Geometry: final body of the model. Coordinates: model frame, mm. Face numbers are marked on the shaded views. A direction names the side the tool comes from. Give positions to 0.01 mm unless a question says otherwise; leave off trailing zeros. Write each loop counter-clockwise with the first axis right and the second up, starting at its lowest first coordinate (ties: lowest second). Pieces come first, ordered by that corner, then holes. Notation, with made-up numbers: M -37.5,-15 L 12.5,-15 A22 cw 12.5,-1 Z; hole C 45.25,-14.5 d7. An arc over 180 degrees is marked long. Use a Markdown table: item, result. Add a question column.
(1) Pin query (flat end, axial travel): pin 1 Ø0.9 at (x, z) = (16.5, 5.5) entering from -Y; pin 2 Ø6 at (x, y) = (12.5, 1) entering from +Z (3 decimals); pin 3 Ø8 at (x, y) = (-6.5, 0) entering from +Z; pin 4 Ø8.5 at (x, y) = (9, 0) entering from +Z. Return the tip coordinate at first contact, or that it passes through.
(2) Material intervals for L1, parallel to Y at x = 9, z = 1; L2, parallel to X at y = -2, z = 3.25 (3 decimals); L3, parallel to Z at x = -6, y = 5, sorted ascending.
(3) Cut plane B-B (z = 4.25). Output: boundary loops of the cut face in (x, y) (3 decimals).
(4) Draft query along X for the marked faces 4, 5 and 6. Return one class per face: released by +X, released by -X, zero draft, split by the parting line, or undercut.
(5) Cut plane C-C (x = 9). Output: boundary loops of the cut face in (y, z).
(6) Cut plane D-D (y = 2.5). Output: boundary loops of the cut face in (x, z) (3 decimals).
(7) Reachability of the marked faces 1, 2 and 3 from +Z, -Z, +X, -X, +Y, -Y: full face, straight path, thin tool, end or side. Return the list, or none.
(8) Cut plane A-A (y = 0). Output: boundary loops of the cut face in (x, z) (3 decimals).
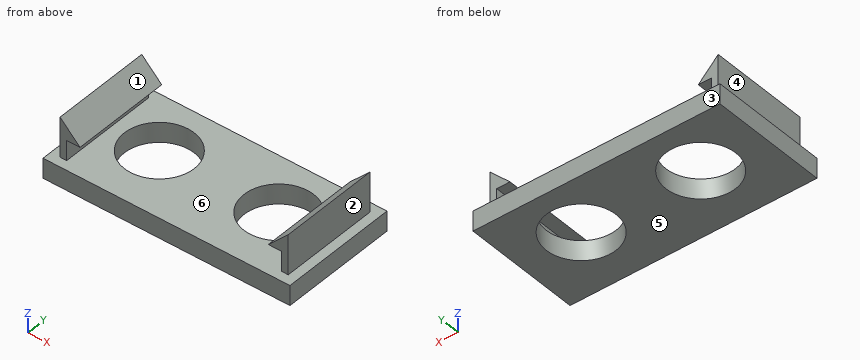
Autodesk Inventor part; units mm, degrees
ref_plane "YZ Plane" through (0, 0, 0) normal (1, 0, 0) x (0, 1, 0)
ref_plane "XZ Plane" through (0, 0, 0) normal (0, 1, 0) x (-1, 0, 0)
ref_plane "XY Plane" through (0, 0, 0) normal (0, 0, 1) x (1, 0, 0)
sketch "Sketch1" plane through (0, 0, 0) normal (0, 0, 1) x (1, 0, 0)
  circle A0 centre (-9, 0) radius 5.25
  circle A1 centre (9, 0) radius 5.25
  line L0 (-16.175, 6.75) -> (16.175, 6.75)
  line L1 (-16.175, -8.25) -> (-16.175, 6.75)
  line L2 (16.175, -8.25) -> (-16.175, -8.25)
  line L3 (16.175, 6.75) -> (16.175, -8.25)
  line L4 (-16.175, 6.75) -> (16.175, -8.25) construction
  line L5 (16.175, 6.75) -> (-16.175, -8.25) construction
  point P0 (0, 0)
  point P1 (0, -7.6531)
  point P2 (14.6494, -5.75)
  point P3 (0, -0.75)
  dimension "d2" = 10.5
  dimension "d3" = 32.35
  dimension "d4" = 32.35
  dimension "d5" = 16.175
  dimension "d6" = 15
  dimension "d7" = 15
  dimension "d8" = 12.5
  dimension "d9" = 18
  dimension "d12" = 9
  dimension "d13" = 9
  dimension "d14" = 10.5
  dimension "d15" = 6.75
  dimension "d16" = 6.75
extrude "Extrusion1" add sketch "Sketch1" along normal blind 3
sketch "Sketch2" plane through (0, 0, 0) normal (0, 0, -1) x (-1, 0, 0)
  circle A0 centre (-9, 0) radius 5.25
  circle A1 centre (9, 0) radius 5.25
  line L0 (-16.175, 6.75) -> (16.175, 6.75)
  line L1 (-16.175, -8.25) -> (-16.175, 6.75)
  line L2 (16.175, -8.25) -> (-16.175, -8.25)
  line L3 (16.175, 6.75) -> (16.175, -8.25)
  line L4 (-16.175, 6.75) -> (-17.175, 6.75)
  line L5 (-17.175, 6.75) -> (-17.175, -8.25)
  line L6 (-17.175, -8.25) -> (-16.175, -8.25)
  line L7 (-16.175, -8.25) -> (-16.175, 6.75)
  line L8 (16.175, 6.75) -> (17.175, 6.75)
  line L9 (17.175, 6.75) -> (17.175, -8.25)
  line L10 (17.175, -8.25) -> (16.175, -8.25)
  line L11 (16.175, -8.25) -> (16.175, 6.75)
  point P0 (0, 0)
  dimension "d17" = 1
  dimension "d18" = 1
extrude "Extrusion2" add sketch "Sketch2" against normal blind 6 contours L1 L6 L5 L4 | L8 L9 L10 L3
sketch "Sketch3" plane through (-17.175, -8.25, 0) normal (0, -1, 0) x (1, 0, 0)
  line L0 (0, 6) -> (3, 6)
  line L1 (3, 6) -> (0, 9)
  line L2 (0, 9) -> (0, 6)
  line L3 (34.35, 6) -> (31.35, 6)
  line L4 (34.35, 6) -> (33.35, 6)
  line L5 (31.35, 6) -> (34.35, 9)
  line L6 (34.35, 9) -> (34.35, 6)
  point P0 (17.175, 0)
  dimension "d21" = 45
  dimension "d22" = 3
  dimension "d23" = 45
  dimension "d35" = 3
extrude "Extrusion3" add sketch "Sketch3" against normal blind 15
sketch "Sketch4" plane through (0, 0, 0) normal (0, 0, -1) x (-1, 0, 0)
  circle A0 centre (-9, 0) radius 5.25
  circle A1 centre (9, 0) radius 5.25
  line L0 (-17.175, 6.75) -> (17.175, 6.75)
  line L1 (-17.175, 6.75) -> (-17.175, -8.25)
  line L2 (-17.175, -8.25) -> (17.175, -8.25)
  line L3 (17.175, -8.25) -> (17.175, 6.75)
  line L4 (17.175, -8.25) -> (18.5892, -9.6642)
  line L5 (17.175, -8.25) -> (19.175, -8.25) construction
  line L6 (17.175, 6.75) -> (18.5892, 8.1642)
  line L7 (17.175, 6.75) -> (19.175, 6.75) construction
  line L8 (-17.175, 6.75) -> (-18.5892, 8.1642)
  line L9 (-17.175, 6.75) -> (-15.175, 6.75) construction
  line L10 (-17.175, 6.75) -> (-17.175, -8.25)
  line L11 (-18.5892, 8.1642) -> (18.5892, 8.1642)
  line L12 (18.5892, -9.6642) -> (18.5892, 8.1642)
  line L13 (18.5892, -9.6642) -> (-18.5892, -9.6642)
  line L14 (18.5892, -9.6642) -> (55.7676, -9.6642) construction
  line L15 (-18.5892, -9.6642) -> (-18.5892, 8.1642)
  point P0 (0, 0)
  dimension "d26" = 2
  dimension "d27" = 45
  dimension "d28" = 2
  dimension "d29" = 45
  dimension "d30" = 2
  dimension "d31" = 135
  dimension "d32" = 180
extrude "Extrusion4" add sketch "Sketch4" against normal blind 3 contours L8 L11 L6 L0 | L1 L2 L4 L13 L15 L8 | L6 L12 L4 L3
equation "\"d4\" = d3"
equation "\"d7\" = d6"
equation "\"d14\" = d2"
Answer list:
| question | item | result |
|---|---|---|
| 1 | pin 1 | y = -8.25 |
| 1 | pin 2 | z = 7.325 |
| 1 | pin 3 | z = 3 |
| 1 | pin 4 | through |
| 2 | L1 | -9.66 to -5.25, 5.25 to 8.16 |
| 2 | L2 | -17.175 to -16.175, 16.175 to 17.175 |
| 2 | L3 | 0 to 3 |
| 3 | outline | M -17.175,-8.25 L -16.175,-8.25 L -16.175,6.75 L -17.175,6.75 Z; M 16.175,-8.25 L 17.175,-8.25 L 17.175,6.75 L 16.175,6.75 Z |
| 4 | face 4 | released by -X |
| 4 | face 5 | zero draft |
| 4 | face 6 | undercut |
| 5 | outline | M -9.66,0 L -5.25,0 L -5.25,3 L -9.66,3 Z; M 5.25,0 L 8.16,0 L 8.16,3 L 5.25,3 Z |
| 6 | outline | M -18.589,0 L -13.617,0 L -13.617,3 L -16.175,3 L -16.175,6 L -14.175,6 L -17.175,9 L -17.175,3 L -18.589,3 Z; M -4.383,0 L 4.383,0 L 4.383,3 L -4.383,3 Z; M 13.617,0 L 18.589,0 L 18.589,3 L 17.175,3 L 17.175,9 L 14.175,6 L 16.175,6 L 16.175,3 L 13.617,3 Z |
| 7 | face 1 | +Z, +Y, -Y |
| 7 | face 2 | +Z, +X, +Y, -Y |
| 7 | face 3 | +Z, -Z, +X, -X, +Y |
| 8 | outline | M -18.589,0 L -14.25,0 L -14.25,3 L -16.175,3 L -16.175,6 L -14.175,6 L -17.175,9 L -17.175,3 L -18.589,3 Z; M -3.75,0 L 3.75,0 L 3.75,3 L -3.75,3 Z; M 14.175,6 L 16.175,6 L 16.175,3 L 14.25,3 L 14.25,0 L 18.589,0 L 18.589,3 L 17.175,3 L 17.175,9 Z |
